Source: CAD feature listing. Evaluate the final solid. Frame: model axes, mm. A direction names the side the tool comes from. Give positions to 0.01 mm unless a question says otherwise; leave off trailing zeros. Order: outer loops, then holes, each group sorted by start corner. A loop starts at its lowest first (then second) coordinate and runs counter-clockwise, first axis right, second up. Notation, with made-up numbers: (50, -20.75) -> (108, -20.75) arc R26 cw to (108, 3.25) -> close; hole circle Ø6 at (-28.5, 34.25). An arc over 180 degrees is marked (long way). Answer in a Markdown table with one row per item.
```python
from build123d import *

# Parameters (mm, degrees)
CONG_1_R = 3


with BuildPart() as part:
    # Esquisse1 → Révolution1 (revolve)
    with BuildSketch(Plane.XY):
        Polygon((-2.65, 0), (-12.5, 0), (-12.5, 7.6), (-4.9, 7.6), (-4.9, 2.6), (-2.65, 2.6), align=None)
    revolve(axis=Axis((0, 17.675608337, 0), (0, -1, 0)))

    # Congé1
    cong_1_edges = [part.edges().sort_by_distance(p)[0] for p in [
        (12.5, 7.6, 0),
    ]]
    fillet(cong_1_edges, radius=CONG_1_R)


solid = part.part
```
(1) Ray query, probe 1 along X at (y, z) = (3.95, 0); probe 2 along X at (y, z) = (1.7, 0). Return the intervals inside material, ascending.
A:
| item | result |
|---|---|
| probe 1 | x = -12.5 to -4.9, 4.9 to 12.5 |
| probe 2 | x = -12.5 to -2.65, 2.65 to 12.5 |
(2) Section query B-B (z = 0). Return the cut outline in (x, y), plus the area to 3 significant figures.
A:
| item | result |
|---|---|
| outline | (-12.5, 0) -> (-2.65, 0) -> (-2.65, 2.6) -> (-4.9, 2.6) -> (-4.9, 7.6) -> (-9.5, 7.6) arc R3 ccw to (-12.5, 4.6) -> close; (2.65, 0) -> (12.5, 0) -> (12.5, 4.6) arc R3 ccw to (9.5, 7.6) -> (4.9, 7.6) -> (4.9, 2.6) -> (2.65, 2.6) -> close |
| area | 123 mm^2 |
(3) Section query A-A (x = 0). Return the cut outline in (y, z), plus the area to 3 significant figures.
A:
| item | result |
|---|---|
| outline | (0, -12.5) -> (4.6, -12.5) arc R3 ccw to (7.6, -9.5) -> (7.6, -4.9) -> (2.6, -4.9) -> (2.6, -2.65) -> (0, -2.65) -> close; (0, 2.65) -> (2.6, 2.65) -> (2.6, 4.9) -> (7.6, 4.9) -> (7.6, 9.5) arc R3 ccw to (4.6, 12.5) -> (0, 12.5) -> close |
| area | 123 mm^2 |
(4) Pull-direction query (Z, two-part tool) for faces 1 (the flat face through (-4, 7.6, 4)), 2 (the cylindrical face through (-11.923, 2.332, -3.755)), 3 (the cylindrical face through (-2.45, 1.28, 1.01)); classes: +Z half, -Z half, draft (parallel to the pull), parting line (faces both ways), or undercut.
A:
| item | result |
|---|---|
| face 1 | draft |
| face 2 | parting line |
| face 3 | undercut |
(5) First-contact query: pin 1 Ø11 at (x, z) = (-2, -2) entering from +Y; pin 2 Ø9 at (x, z) = (0, 0) entering from +Y; pin 3 Ø4 at (y, z) = (4, 3) entering from +X; pin 4 Ø1 at (y, z) = (5.5, -1.5) entering from -X. Flat tips, straight axial feed; report the tip coordinate or a pass-through.
A:
| item | result |
|---|---|
| pin 1 | stops at y = 7.6 |
| pin 2 | stops at y = 2.6 |
| pin 3 | stops at x = 12.46 |
| pin 4 | stops at x = -12.4 |
(6) Access query for faces 4 (the cylindrical face through (1.062, 5.065, 4.783)), 5 (the flat face through (0, 0, -3)). Directions: +Z, -Z, +X, -X, +Y, -Y. A direction counts if a zero-diameter tool reaches every point of the face in a straight line with its end or side. Return the directions, or none.
A:
| item | result |
|---|---|
| face 4 | +Y |
| face 5 | +Z, -Z, +X, -X, -Y |
(7) Section query C-C (y = 4). Return the cut outline in (x, z), plus the area to 3 significant figures.
A:
| item | result |
|---|---|
| outline | circle Ø25 at (0, 0); hole circle Ø9.8 at (0, 0) |
| area | 415 mm^2 |
